For this review, take the finished solid that the model builds, in its own axes (mm). Round coordinates to 2 decimals unless told otherwise and drop trailing zeros. Loops run counter-clockwise (first coordinate to the right, second up) from the corner with the lowest first, then second, coordinate; pieces in that order, holes last. Notation, with made-up numbers: (-13.75, -12.75) -> (43.25, -12.75) arc R35 ccw to (43.25, 22.25) -> close; hole circle Ø9 at (-24, 2). An arc over 180 degrees is marked (long way). Write each question's results on one line, items separated by ' | '.
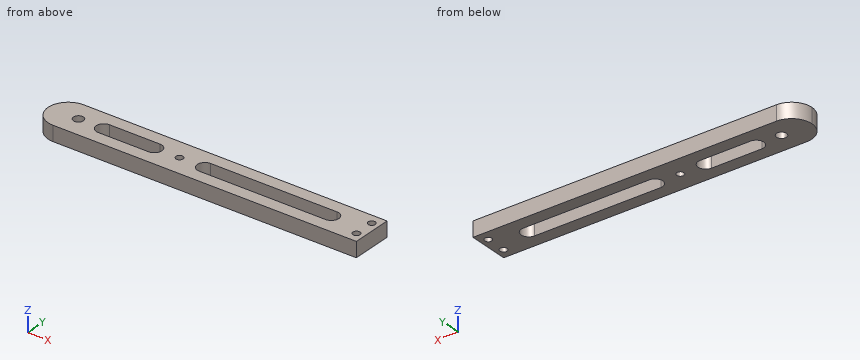
```python
from build123d import *

# Parameters (mm, degrees)
SKETCH1_W                 = 203.2
SKETCH1_H                 = 25.4
BOSS_EXTRUDE1_DEPTH       = 9.525
F_8_CLEARANCE_HOLE1_D     = 4.4958
F_8_CLEARANCE_HOLE1_DEPTH = 25.4
F_8_CLEARANCE_HOLE1_TIP   = 1.350674586
SKETCH5_R                 = 3.1623
CUT_EXTRUDE1_DEPTH        = 9.525
F_8_CLEARANCE_HOLE2_D     = 4.4958
F_8_CLEARANCE_HOLE2_DEPTH = 19.05
F_8_CLEARANCE_HOLE2_TIP   = 1.350674586
CUT_EXTRUDE2_DEPTH        = 10.525
CUT_EXTRUDE3_DEPTH        = 10.525


with BuildPart() as part:
    # Sketch1 → Boss-Extrude1 (new body)
    with BuildSketch(Plane.XY):
        with Locations((-101.6, 12.7)):
            Rectangle(SKETCH1_W, SKETCH1_H)
    extrude(amount=BOSS_EXTRUDE1_DEPTH)

    # #8 Clearance Hole1
    with Locations(Plane.XY.offset(9.525)):
        with Locations((-4.7625, 6.35), (-4.7625, 19.05)):
            Hole(F_8_CLEARANCE_HOLE1_D / 2, depth=F_8_CLEARANCE_HOLE1_DEPTH)
            with Locations((0, 0, -(F_8_CLEARANCE_HOLE1_DEPTH + F_8_CLEARANCE_HOLE1_TIP / 2))):  # 118° drill point
                Cone(0, F_8_CLEARANCE_HOLE1_D / 2, F_8_CLEARANCE_HOLE1_TIP, mode=Mode.SUBTRACT)

    # Sketch5 → Cut-Extrude1 (cut)
    with BuildSketch(Plane.XY.offset(9.525)):
        with Locations((-184.15, 12.7)):
            Circle(SKETCH5_R)
    extrude(amount=-CUT_EXTRUDE1_DEPTH, mode=Mode.SUBTRACT)

    # #8 Clearance Hole2
    with Locations(Plane.XY.offset(9.525)):
        with Locations((-120.65, 12.7)):
            Hole(F_8_CLEARANCE_HOLE2_D / 2, depth=F_8_CLEARANCE_HOLE2_DEPTH)
            with Locations((0, 0, -(F_8_CLEARANCE_HOLE2_DEPTH + F_8_CLEARANCE_HOLE2_TIP / 2))):  # 118° drill point
                Cone(0, F_8_CLEARANCE_HOLE2_D / 2, F_8_CLEARANCE_HOLE2_TIP, mode=Mode.SUBTRACT)

    # Sketch10 → Cut-Extrude2 (cut, through all)
    with BuildSketch(Plane.XY.offset(9.525)):
        with BuildLine():
            Line((-190.5, 25.4), (-203.2, 25.4))
            Line((-203.2, 25.4), (-203.2, 12.7))
            ThreePointArc((-203.2, 12.7), (-199.480256121, 21.680256121), (-190.5, 25.4))
        make_face()
        with BuildLine():
            ThreePointArc((-190.5, 0), (-199.480256121, 3.719743879), (-203.2, 12.7))
            Line((-203.2, 12.7), (-203.2, 0))
            Line((-203.2, 0), (-190.5, 0))
        make_face()
    extrude(amount=-CUT_EXTRUDE2_DEPTH, mode=Mode.SUBTRACT)

    # Sketch11 → Cut-Extrude3 (cut, through all)
    with BuildSketch(Plane(origin=(0, 0, 0), x_dir=(-1, 0, 0), z_dir=(0, 0, -1))):
        with BuildLine():
            Line((25.4, 17.4625), (104.775, 17.4625))
            ThreePointArc((104.775, 17.4625), (109.5375, 12.7), (104.775, 7.9375))
            Line((104.775, 7.9375), (25.4, 7.9375))
            ThreePointArc((25.4, 7.9375), (20.6375, 12.7), (25.4, 17.4625))
        make_face()
        with BuildLine():
            Line((136.525, 17.4625), (168.275, 17.4625))
            ThreePointArc((168.275, 17.4625), (173.0375, 12.7), (168.275, 7.9375))
            Line((168.275, 7.9375), (136.525, 7.9375))
            ThreePointArc((136.525, 7.9375), (131.7625, 12.7), (136.525, 17.4625))
        make_face()
    extrude(amount=-CUT_EXTRUDE3_DEPTH, mode=Mode.SUBTRACT)


solid = part.part
```
1. Consider section D-D (y = 2). State the section outline as (x, z) points (3 decimals), plus the area to 3 significant figures.
Values found:
outline: (-197.341, 0) -> (0, 0) -> (0, 9.525) -> (-197.341, 9.525) -> close | area: 1,880 mm2
2. Consider section C-C (x = -184.15). State the section outline as (y, z) points (3 decimals).
Values found:
outline: (0, 0) -> (9.538, 0) -> (9.538, 9.525) -> (0, 9.525) -> close; (15.862, 0) -> (25.4, 0) -> (25.4, 9.525) -> (15.862, 9.525) -> close
3. Consider section B-B (z = 6.5). Give the number of separate pieces and of enclosed holes in the cut face, plus the area to 3 significant figures.
Values found:
separate pieces: 1 | enclosed holes: 6 | area: 3,810 mm2
4. For pin 1 (2.5 mm diameter, centred on x = -4.76, y = 6.35, fed in from -Z), flat-tipped, find the tip position at first contact; note if it passes through.
Values found:
pin 1: passes through
5. To check wall thickness, follow probe 1 along X at (y, z) = (12.5, 1.75); probe 2 along Y at (x, z) = (-95, 4.75); probe 3 along Y at (x, z) = (-120.65, 2). State the ranges of each line that lie inside material, in increasing order.
Values found:
probe 1: x = -203.2 to -187.31, -180.99 to -173.03, -131.77 to -122.89, -118.41 to -109.53, -20.64 to 0 | probe 2: y = 0 to 7.94, 17.46 to 25.4 | probe 3: y = 0 to 10.45, 14.95 to 25.4
6. Consider section A-A (x = -59.5). State the section outline as (y, z) points (1 decimal), plus the area to 3 significant figures.
Values found:
outline: (0, 0) -> (7.9, 0) -> (7.9, 9.5) -> (0, 9.5) -> close; (17.5, 0) -> (25.4, 0) -> (25.4, 9.5) -> (17.5, 9.5) -> close | area: 151 mm2
